Geometry check sheet. Reference: the model listing, model coordinates, mm. Face numbers are marked on the shaded views. Give positions to 0.01 mm unless a question says otherwise; leave off trailing zeros. Write each loop counter-clockwise with the first axis right and the second up, starting at its lowest first coordinate (ties: lowest second). Pieces come first, ordered by that corner, then holes. Notation, with made-up numbers: (-17, 70) - (6, 70) arc R21 cw to (6, 84) - close; hole circle Ø7 at (-5, 85.25). An arc over 180 degrees is marked (long way). Use a Markdown table: item, result.
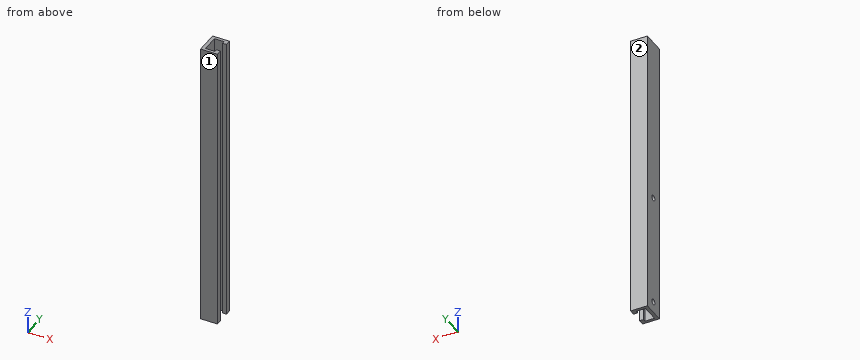
```python
from build123d import *

# Parameters (mm, degrees)
BOSS_EXTRUDE1_DEPTH = 660.4
SKETCH2_R           = 6.35
CUT_EXTRUDE1_DEPTH  = 38.944489796


with BuildPart() as part:
    # Sketch1 → Boss-Extrude1 (new body)
    with BuildSketch(Plane.XY):
        Polygon((13.996027612, 10.491268563), (22.704599041, 10.491268563), (22.704599041, 23.093265306), (-15.239890755, 23.093265306), (-15.239890755, -27.706734694), (22.704599041, -27.706734694), (22.704599041, -15.006734694), (13.996027612, -15.006734694), (13.996027612, -21.356734694), (-7.619890755, -21.356734694), (-7.619890755, 16.743265306), (13.996027612, 16.743265306), align=None)
    extrude(amount=BOSS_EXTRUDE1_DEPTH)

    # Sketch2 → Cut-Extrude1 (cut, through all)
    with BuildSketch(Plane.ZY.offset(15.239890755)):
        with Locations((25.4, -2.306734694)):
            Circle(SKETCH2_R)
        with Locations((279.4, -2.306734694)):
            Circle(SKETCH2_R)
    extrude(amount=-CUT_EXTRUDE1_DEPTH, mode=Mode.SUBTRACT)


solid = part.part
```
1) Depth check by flat-ended pin: P1, Ø8, axis at x = -0.5, y = 13.5, coming from the -Z side; P2, Ø7.5, axis at y = -2.31, z = 25.4, coming from the +X side. Enter the tip coordinate at first touch or a pass-through.
Working result:
| item | result |
|---|---|
| P1 | stops at z = 0 |
| P2 | passes through |
2) Section check C-C on z = 564.5. Record the boundary of the cut face in (x, y).
Working result:
| item | result |
|---|---|
| outline | (-15.24, -27.71) - (22.7, -27.71) - (22.7, -15.01) - (14, -15.01) - (14, -21.36) - (-7.62, -21.36) - (-7.62, 16.74) - (14, 16.74) - (14, 10.49) - (22.7, 10.49) - (22.7, 23.09) - (-15.24, 23.09) - close |
3) Mould release check, pull along Y, two halves, no side actions. Record for the marked faces 1 and 2: pulls with the +Y half, pulls with the -Y half, needs draft (parallel to the pull), parting line crosses it, or undercut.
Working result:
| item | result |
|---|---|
| face 1 | pulls with the -Y half |
| face 2 | pulls with the +Y half |
4) Section check B-B on x = -0.5. Record the boundary of the cut face in (y, z), then the cut area to 3 significant figures.
Working result:
| item | result |
|---|---|
| outline | (-27.71, 0) - (-21.36, 0) - (-21.36, 660.4) - (-27.71, 660.4) - close; (16.74, 0) - (23.09, 0) - (23.09, 660.4) - (16.74, 660.4) - close |
| area | 8,390 mm² |
5) Section check A-A on z = 279.4. Record the boundary of the cut face in (x, y), then the cut area to 3 significant figures.
Working result:
| item | result |
|---|---|
| outline | (-15.24, -27.71) - (22.7, -27.71) - (22.7, -15.01) - (14, -15.01) - (14, -21.36) - (-7.62, -21.36) - (-7.62, -8.66) - (-15.24, -8.66) - close; (-15.24, 4.04) - (-7.62, 4.04) - (-7.62, 16.74) - (14, 16.74) - (14, 10.49) - (22.7, 10.49) - (22.7, 23.09) - (-15.24, 23.09) - close |
| area | 785 mm² |
6) Material ranges on L1, parallel to Y at x = -12, z = 25; L2, parallel to X at y = -18, z = 382.5; L3, parallel to Y at x = 6, z = 35, recorded low to high. Write a range as from..to.
Working result:
| item | result |
|---|---|
| L1 | y = -27.71..-8.64, 4.03..23.09 |
| L2 | x = -15.24..-7.62, 14..22.7 |
| L3 | y = -27.71..-21.36, 16.74..23.09 |
